```python
from build123d import *

# Parameters (mm, degrees)
SKETCH_R     = 1.5
PAD_DEPTH    = 5
SKETCH001_W  = 3
SKETCH001_H  = 8
PAD001_DEPTH = 8
SKETCH002_R  = 1.5
POCKET_DEPTH = 23


with BuildPart() as part:
    # Sketch → Pad (new body)
    with BuildSketch(Plane.XY):
        with BuildLine():
            Line((32.750175, 18.812472), (62.750175, 18.812472))
            ThreePointArc((62.750169, 10.812472), (66.750155, 14.812469), (62.750175, 18.812472))
            Line((32.750169, 10.812472), (62.750169, 10.812472))
            ThreePointArc((32.750175, 18.812472), (28.750176, 14.812476), (32.750169, 10.812472))
        make_face()
        with Locations((32.750176, 14.812472)):
            Circle(SKETCH_R, mode=Mode.SUBTRACT)
        with Locations((62.750155, 14.812472)):
            Circle(SKETCH_R, mode=Mode.SUBTRACT)
        with Locations((50.750155, 14.812472)):
            Circle(SKETCH_R, mode=Mode.SUBTRACT)
        with Locations((44.750176, 14.812472)):
            Circle(SKETCH_R, mode=Mode.SUBTRACT)
    extrude(amount=PAD_DEPTH)

    # Sketch001 (on Face10 of Pad) → Pad001 (join)
    with BuildSketch(Plane.XY.offset(5)):
        with Locations((39.250176, 14.812472)):
            Rectangle(SKETCH001_W, SKETCH001_H)
        with Locations((56.250155, 14.788555)):
            Rectangle(SKETCH001_W, SKETCH001_H)
    extrude(amount=PAD001_DEPTH)

    # Sketch002 (on Face20 of Pad001) → Pocket (cut)
    with BuildSketch(Plane.YZ.offset(57.750155)):
        with Locations((14.788555, 9.5)):
            Circle(SKETCH002_R)
    extrude(amount=-POCKET_DEPTH, mode=Mode.SUBTRACT)


solid = part.part
```
Check sheet for the modelled part. Datum: model origin and axes. Units: mm. A direction names the side the tool comes from. Round coordinates to 2 decimals unless told otherwise and drop trailing zeros. Loops run counter-clockwise (first coordinate to the right, second up) from the corner with the lowest first, then second, coordinate; pieces in that order, holes last. Notation, with made-up numbers: (83, 15) -> (101, 15) arc R12 cw to (101, 31) -> close; hole circle Ø3 at (-34, 17). An arc over 180 degrees is marked (long way). Write item = value, one per line. Start each with the question number.
1) Sectioned sample at C-C, the plane x = 58.5. Record the cut outline in (y, z).
2) Gauge pin test, flat ends, axial feed: pin 1 Ø4 at (y, z) = (14.79, 9.5) entering from -X; pin 2 Ø3.5 at (x, y) = (44.75, 14.81) entering from +Z; pin 3 Ø2.5 at (x, y) = (50.75, 14.81) entering from -Z; pin 4 Ø2.5 at (y, z) = (16, 7.5) entering from +X. Record the tip position at first contact, or that the pin passes through.
3) Release check for a two-part mould opening along Y. For faces 1 (the cylindrical face through (61.56, 13.9, 2.46)), 2 (the flat face through (40.75, 14, 8)), 3 (the cylindrical face through (66.75, 14.72, 2.46)), 4 (the cylindrical face through (43.56, 13.9, 2.46)) record: released by +Y, released by -Y, zero draft, split by the parting line, or undercut.
4) Set-up check for faces 5 (the flat face through (34.3, 14, 5)), 6 (the flat face through (54.75, 14, 8)): record each of +Z, -Z, +X, -X, +Y, -Y from which the full face is reachable in a straight line by a thin tool's end or side.
5) Sectioned sample at B-B, the plane z = 11.75. Record the cut outline in (x, y).
6) Thickness scan on probe 1 along X at (y, z) = (13.75, 7.25); probe 2 along X at (y, z) = (15.5, 1); probe 3 along Y at (x, z) = (59, 3). Record the ranges inside material, lowest first.
7) Sectioned sample at A-A, the plane z = 9.5. Record the cut outline in (x, y).
8) Sectioned sample at D-D, the plane y = 12. Record the cut outline in (x, z), plus the area to 3 significant figures.
Results are:
q1.outline = (10.81, 0) -> (18.81, 0) -> (18.81, 5) -> (10.81, 5) -> close
q2.pin_1 = 37.75
q2.pin_2 = 5
q2.pin_3 = through
q2.pin_4 = 57.75
q3.face_1 = undercut
q3.face_2 = zero draft
q3.face_3 = split by the parting line
q3.face_4 = undercut
q4.face_5 = +Z, -X, +Y, -Y
q4.face_6 = +Z, +Y, -Y
q5.outline = (37.75, 10.81) -> (40.75, 10.81) -> (40.75, 18.81) -> (37.75, 18.81) -> close; (54.75, 10.79) -> (57.75, 10.79) -> (57.75, 18.79) -> (54.75, 18.79) -> close
q6.probe_1 = 37.75 to 40.75, 54.75 to 57.75
q6.probe_2 = 28.81 to 31.42, 34.08 to 43.42, 46.08 to 49.42, 52.08 to 61.42, 64.08 to 66.69
q6.probe_3 = 10.81 to 18.81
q7.outline = (37.75, 10.81) -> (40.75, 10.81) -> (40.75, 13.29) -> (37.75, 13.29) -> close; (37.75, 16.29) -> (40.75, 16.29) -> (40.75, 18.81) -> (37.75, 18.81) -> close; (54.75, 10.79) -> (57.75, 10.79) -> (57.75, 13.29) -> (54.75, 13.29) -> close; (54.75, 16.29) -> (57.75, 16.29) -> (57.75, 18.79) -> (54.75, 18.79) -> close
q8.outline = (29.91, 0) -> (65.59, 0) -> (65.59, 5) -> (57.75, 5) -> (57.75, 13) -> (54.75, 13) -> (54.75, 5) -> (40.75, 5) -> (40.75, 13) -> (37.75, 13) -> (37.75, 5) -> (29.91, 5) -> close
q8.area = 226 mm^2
